Read the model definition and answer for the solid it produces. Units are mm, in the model's axes. Face numbers are marked on the shaded views. Round coordinates to 2 decimals unless told otherwise and drop trailing zeros. Loops run counter-clockwise (first coordinate to the right, second up) from the corner with the lowest first, then second, coordinate; pieces in that order, holes last. Notation, with made-up numbers: (18, 77) - (46, 77) arc R19 ccw to (46, 103) - close; hole circle Ø8 at (39.5, 84). An arc over 180 degrees is marked (long way). Use CSV: the item, a comma, the result in double quotes. Start each with the question number.
1. Determine the mould class of the marked faces 1, 2 and 3 for opening direction Z: +Z half, -Z half, draft (parallel to the pull), parting line (faces both ways), or undercut.
2. Find section C-C (x = 13.5). Give the vertices of the cut face in (y, z).
3. Find section A-A (y = 2.5). Give the vertices of the cut face in (x, z).
4. Find section D-D (z = 14.5). Give the vertices of the cut face in (x, y).
5. Given pin 1 Ø1.5 at (x, z) = (44.5, 17.5) entering from +Y; pin 2 Ø8 at (x, z) = (4.5, -19) entering from +Y; pin 3 Ø0.6 at (x, z) = (53, 0.5) entering from +Y, each flat-ended and moving along its own axis, determine where each tip first touches the part or whether it passes through.
6. Consider line 1 along X through (y, z) = (3, 0); line 2 along X through (y, z) = (8.25, 0); line 3 along Z through (x, y) = (0, 3.25). Determine where each line is inside the solid, lowest interval first.
7. Find section B-B (x = 25.4). Give the vertices of the cut face in (y, z).
from build123d import *

# Parameters (mm, degrees)
SKETCH1_W           = 91
SKETCH1_H           = 62
SKETCH1_R           = 6
BOSS_EXTRUDE1_DEPTH = 6
SKETCH16_W          = 3
SKETCH16_H          = 10
SKETCH16_W_2        = 10
SKETCH16_R          = 3
BOSS_EXTRUDE3_DEPTH = 4
SKETCH16_4_R        = 3
BOSS_EXTRUDE4_DEPTH = 10
FILLET1_R           = 2
BOSS_EXTRUDE5_DEPTH = 91
SKETCH1_2_R         = 6
CUT_EXTRUDE1_DEPTH  = 12


with BuildPart() as part:
    # Sketch1 → Boss-Extrude1 (new body)
    with BuildSketch(Plane(origin=(0, 0, 0), x_dir=(1, 0, 0), z_dir=(0, 1, 0))):
        Rectangle(SKETCH1_W, SKETCH1_H)
        with Locations((-25.4, 0)):
            Circle(SKETCH1_R, mode=Mode.SUBTRACT)
        Circle(SKETCH1_R, mode=Mode.SUBTRACT)
        with Locations((25.4, 0)):
            Circle(SKETCH1_R, mode=Mode.SUBTRACT)
    extrude(amount=BOSS_EXTRUDE1_DEPTH)

    # Sketch16 → Boss-Extrude3 (add)
    with BuildSketch(Plane.XZ):
        with Locations((47, 0)):
            Rectangle(SKETCH16_W, SKETCH16_H)
        with Locations((53.5, 0)):
            Rectangle(SKETCH16_W_2, SKETCH16_H)
        with Locations((53.5, 0)):
            Circle(SKETCH16_R, mode=Mode.SUBTRACT)
        with Locations((53.5, 0)):
            Circle(SKETCH16_R)
    extrude(amount=-BOSS_EXTRUDE3_DEPTH)

    # Sketch16<4> → Boss-Extrude4 (add)
    with BuildSketch(Plane.XZ):
        with Locations((53.5, 0)):
            Circle(SKETCH16_4_R)
    extrude(amount=-BOSS_EXTRUDE4_DEPTH)

    # Fillet1
    fillet1_edges = [part.edges().sort_by_distance(p)[0] for p in [
        (50.5, 10, 0),
    ]]
    fillet(fillet1_edges, radius=FILLET1_R)

    # Sketch17 → Boss-Extrude5 (add)
    with BuildSketch(Plane.ZY.offset(45.5)):
        with BuildLine():
            Line((-31, 6), (31, 6))
            ThreePointArc((31, 6), (0, 11), (-31, 6))
        make_face()
    extrude(amount=-BOSS_EXTRUDE5_DEPTH)

    # Sketch1<2> → Cut-Extrude1 (cut, through all)
    with BuildSketch(Plane(origin=(0, 0, 0), x_dir=(1, 0, 0), z_dir=(0, 1, 0))):
        with Locations((-25.4, 0)):
            Circle(SKETCH1_2_R)
        Circle(SKETCH1_2_R)
        with Locations((25.4, 0)):
            Circle(SKETCH1_2_R)
    extrude(amount=CUT_EXTRUDE1_DEPTH, mode=Mode.SUBTRACT)


solid = part.part
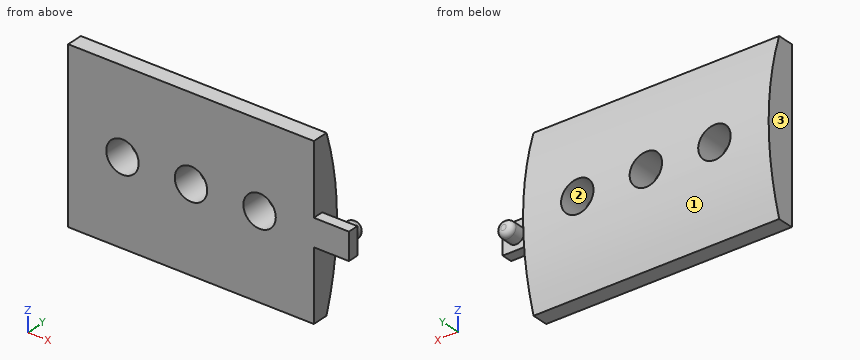
Filled sheet:
1,face 1,"parting line"
1,face 2,"undercut"
1,face 3,"draft"
2,outline,"(0, -31) - (6, -31) arc R98.6 ccw to (6, 31) - (0, 31) - close"
3,outline,"(-45.5, -31) - (45.5, -31) - (45.5, -5) - (58.5, -5) - (58.5, 5) - (45.5, 5) - (45.5, 31) - (-45.5, 31) - close; hole circle Ø12 at (-25.4, 0); hole circle Ø12 at (0, 0); hole circle Ø12 at (25.4, 0)"
4,outline,"(-45.5, 0) - (45.5, 0) - (45.5, 9.93) - (-45.5, 9.93) - close"
5,pin 1,"stops at y = 9.57"
5,pin 2,"stops at y = 9.85"
5,pin 3,"stops at y = 10"
6,line 1,"x = -45.5 to -31.4, -19.4 to -6, 6 to 19.4, 31.4 to 58.5"
6,line 2,"x = -45.5 to -31.4, -19.4 to -6, 6 to 19.4, 31.4 to 45.5, 50.52 to 56.48"
6,line 3,"z = -31 to -6, 6 to 31"
7,outline,"(0, -31) - (6, -31) arc R98.6 ccw to (10.82, -6) - (0, -6) - close; (0, 6) - (10.82, 6) arc R98.6 ccw to (6, 31) - (0, 31) - close"
